```python
from build123d import *

# Parameters (mm, degrees)
CROQUIS1_W              = 54
CROQUIS1_H              = 51
CROQUIS1_R              = 3.75
SALIENTE_EXTRUIR1_DEPTH = 2


with BuildPart() as part:
    # Croquis1 → Saliente-Extruir1 (new body)
    with BuildSketch(Plane.XY):
        Rectangle(CROQUIS1_W, CROQUIS1_H)
        with Locations((-21.5, 12.5)):
            Circle(CROQUIS1_R, mode=Mode.SUBTRACT)
        with Locations((21.5, 12.5)):
            Circle(CROQUIS1_R, mode=Mode.SUBTRACT)
        with Locations((21.5, -9.5)):
            Circle(CROQUIS1_R, mode=Mode.SUBTRACT)
        with Locations((-21.5, -9.5)):
            Circle(CROQUIS1_R, mode=Mode.SUBTRACT)
    extrude(amount=-SALIENTE_EXTRUIR1_DEPTH)


solid = part.part
```
Design review of the part built by this model. Coordinates are the model's own, in mm. Coordinates: 2 decimals unless noted, no trailing zeros. Order: outer loops, then holes, each group sorted by start corner. A loop starts at its lowest first (then second) coordinate and runs counter-clockwise, first axis right, second up. Notation, with made-up numbers: (6.5, 37.25) - (53.5, 37.25) arc R20 ccw to (53.5, 74.25) - close; hole circle Ø9 at (30.25, 33). An arc over 180 degrees is marked (long way). Answer in a Markdown table with one row per item.
(1) The part is to be moulded in two halves that separate along X. For faces 1 (the flat face through (0, 0, -2)), 2 (the flat face through (27, 0, -1)), 3 (the cylindrical face through (23.52, 15.66, -0.99)), say which applies: released by +X, released by -X, zero draft, split by the parting line, or undercut.
Checked values:
| item | result |
|---|---|
| face 1 | zero draft |
| face 2 | released by +X |
| face 3 | undercut |
(2) Wall thickness on line 1 along Y through (x, z) = (21.5, -1.35); line 2 along X through (y, z) = (13.5, -0.85); line 3 along Y through (x, z) = (23, -1.1): over which ranges is each line inside the solid? List them lowest first. Write a range as from..to.
Checked values:
| item | result |
|---|---|
| line 1 | -25.5..-13.25, -5.75..8.75, 16.25..25.5 |
| line 2 | -27..-25.11, -17.89..17.89, 25.11..27 |
| line 3 | -25.5..-12.94, -6.06..9.06, 15.94..25.5 |
(3) Consider section A-A on z = -0.7. State the section outline as (x, y) points, plus the area to 3 significant figures.
Checked values:
| item | result |
|---|---|
| outline | (-27, -25.5) - (27, -25.5) - (27, 25.5) - (-27, 25.5) - close; hole circle Ø7.5 at (-21.5, -9.5); hole circle Ø7.5 at (-21.5, 12.5); hole circle Ø7.5 at (21.5, -9.5); hole circle Ø7.5 at (21.5, 12.5) |
| area | 2,580 mm^2 |
(4) Clearance check with a flat-ended pin moving along its axis: pin 1 (4.5 mm diameter, centred on x = 21.5, y = -9.5, fed in from -Z). State where the tip first meets the part, or that it passes through.
Checked values:
| item | result |
|---|---|
| pin 1 | through |
(5) Consider section B-B on y = 9.5. State the section outline as (x, z) points.
Checked values:
| item | result |
|---|---|
| outline | (-27, -2) - (-23.75, -2) - (-23.75, 0) - (-27, 0) - close; (-19.25, -2) - (19.25, -2) - (19.25, 0) - (-19.25, 0) - close; (23.75, -2) - (27, -2) - (27, 0) - (23.75, 0) - close |
(6) Consider section C-C on x = 19. State the section outline as (y, z) points, plus the area to 3 significant figures.
Checked values:
| item | result |
|---|---|
| outline | (-25.5, -2) - (-12.3, -2) - (-12.3, 0) - (-25.5, 0) - close; (-6.7, -2) - (9.7, -2) - (9.7, 0) - (-6.7, 0) - close; (15.3, -2) - (25.5, -2) - (25.5, 0) - (15.3, 0) - close |
| area | 79.6 mm^2 |
